from build123d import *

# Parameters (mm, degrees)
SKETCH1_R          = 1060
SKETCH1_R_2        = 962
BASE_FLANGE1_DEPTH = 15
SKETCH2_R          = 11
CUT_EXTRUDE1_DEPTH = 20
CIRPATTERN1_COUNT  = 40


# Sheet-metal steps are written as plain solids
with BuildPart() as part:
    # Sketch1 → Base-Flange1 (new body)
    with BuildSketch(Plane.XY):
        Circle(SKETCH1_R)
        Circle(SKETCH1_R_2, mode=Mode.SUBTRACT)
    extrude(amount=-BASE_FLANGE1_DEPTH)

    # Sketch2 → Cut-Extrude1 (cut)
    with BuildSketch(Plane.XY):
        with Locations((79.243686685, 1006.88650707)):
            Circle(SKETCH2_R)
    cut_extrude1 = extrude(amount=-CUT_EXTRUDE1_DEPTH, mode=Mode.SUBTRACT)

    # CirPattern1: Cut-Extrude1 ×40 about axis
    cirpattern1_axis = Axis((0, 0, 0), (0, 0, 1))
    for i in range(1, CIRPATTERN1_COUNT):
        add(cut_extrude1.rotate(cirpattern1_axis, i * 360 / CIRPATTERN1_COUNT), mode=Mode.SUBTRACT)


solid = part.part
The model under review builds one solid part; all positions refer to its coordinate system, in mm. Coordinates: 2 decimals unless noted, no trailing zeros. Write each loop counter-clockwise with the first axis right and the second up, starting at its lowest first coordinate (ties: lowest second). Pieces come first, ordered by that corner, then holes. Notation, with made-up numbers: M 12.5,21 L 41.5,21 A16 cw 41.5,29 Z; hole C 64.5,79 d10. An arc over 180 degrees is marked long. Put each result on its own line as item: value.
1) Add section A-A on y = 0. Give the boundary of the cut face in (x, z), then the cut area to 3 significant figures.
Computed:
outline: M -1060,-15 L -962,-15 L -962,0 L -1060,0 Z; M 962,-15 L 1060,-15 L 1060,0 L 962,0 Z
area: 2,940 mm2
2) Draft analysis for pull direction Y (two halves, no side actions). For faces 1 (the flat face through (-555, 790, -15)), 2 (the cylindrical face through (569.85, 893.796, -7.395)), 3 (the cylindrical face through (443.9, -853.46, -7.4)), state which applies: released by +Y, released by -Y, zero draft, split by the parting line, or undercut.
Computed:
face 1: zero draft
face 2: split by the parting line
face 3: undercut
3) Add section C-C on z = -9. State how many separate pieces and enclosed holes the cut face has, then the cut area to 3 significant figures.
Computed:
separate pieces: 1
enclosed holes: 41
area: 607,000 mm2
4) Wall thickness on probe 1 along Y at (x, z) = (0, -11.5); probe 2 along X at (y, z) = (773, -3); probe 3 along Y at (x, z) = (-661, -3): over which ranges is each line inside the solid? List them lowest first. Write a range as [from, to].
Computed:
probe 1: y = [-1060, -962], [962, 1060]
probe 2: x = [-725.31, -665.75], [-646.14, -572.64], [572.64, 646.14], [665.75, 725.31]
probe 3: y = [-828.66, -777.78], [-758.24, -698.94], [698.94, 758.24], [777.78, 828.66]
5) Clearance check with flat-ended pins moving along their axes: pin 1 Ø17.5 at (x, y) = (-1006.89, 79.24) entering from -Z; pin 2 Ø1.5 at (x, z) = (-314.5, -10.5) entering from +Y; pin 3 Ø1 at (y, z) = (618, -4.5) entering from -X; pin 4 Ø1 at (y, z) = (149.5, -5.5) entering from +X. State where each tip first meets the part, or that it passes through.
Computed:
pin 1: passes through
pin 2: stops at y = 1012.5
pin 3: stops at x = -861.56
pin 4: stops at x = 1049.48
